Study the drawing (mm; zero at the part's minimum x, y, z) and answer. A direction names the side the tool comes from. Coordinates: 2 decimals unless noted, no trailing zeros. Order: outer loops, then holes, each group sorted by start corner. A loop starts at its lowest first (then second) coordinate and runs counter-clockwise, first axis right, second up.
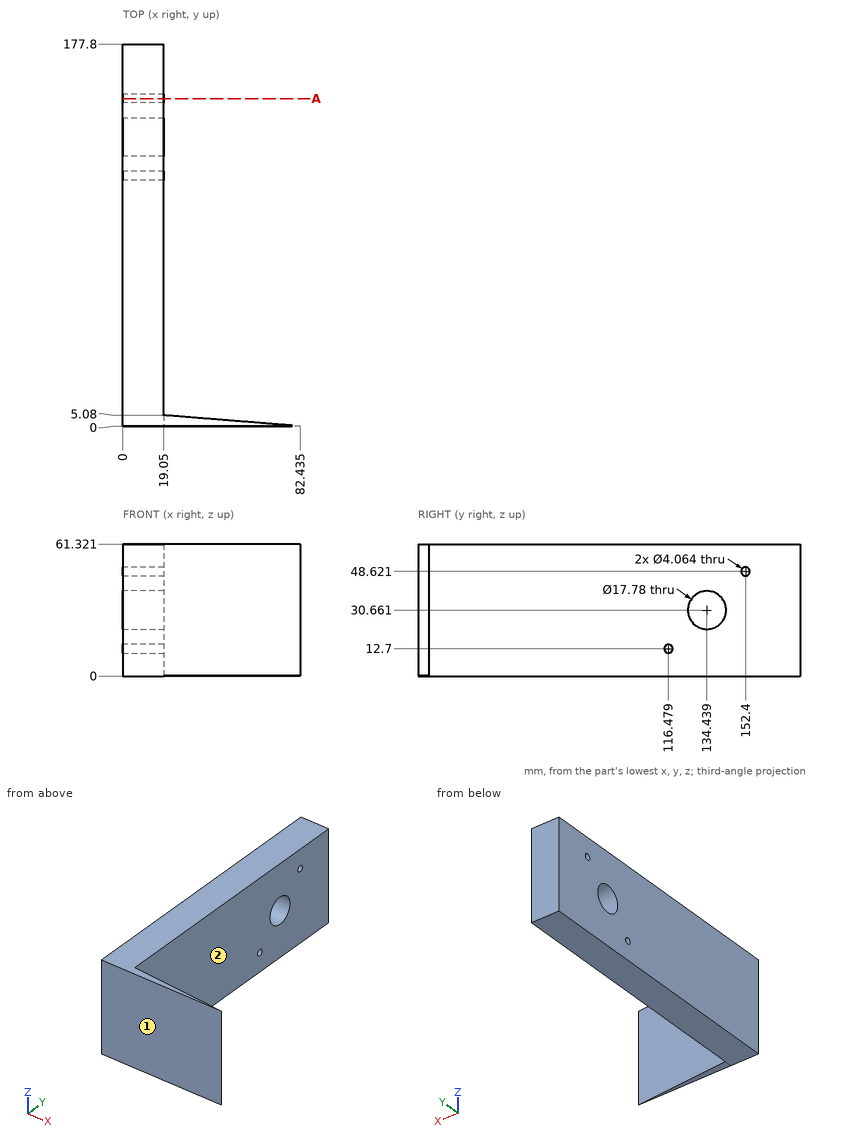
(1) Find section A-A (y = 152.4). Write down the section's boundary in (x, z).
(2) For the marked faces 1 and 2, determine the directions among +Z, -Z, +X, -X, +Y, -Y from which every point of the face is accessible in a straight line to the end or side of a thin tool.
(3) Each of these flat-tipped pins is pushed along its axis until it touches: pin 1 Ø4 at (x, z) = (67.5, 51) entering from -Y; pin 2 Ø3 at (x, z) = (43, 11.5) entering from +Y; pin 3 Ø4.5 at (y, z) = (152.4, 48.62) entering from +X. Where does it stop, or does it pass through?
(4) Consider line 1 (X direction, y = 91, z = 24); line 2 (Z direction, x = 11, y = 152); line 3 (Y direction, x = 4, z = 12) (1 decimal). Determine where each line is inside the solid, lowest interval first.
Findings below:
1. outline: (0, 0) - (19.05, 0) - (19.05, 46.59) - (0, 46.59) - close; (0, 50.65) - (19.05, 50.65) - (19.05, 61.32) - (0, 61.32) - close
2. face 1: +Z, -Z, +X, -X, -Y
2. face 2: +Z, -Z, +X, +Y
3. pin 1: stops at y = 0
3. pin 2: stops at y = 3.28
3. pin 3: stops at x = 19.05
4. line 1: x = 0 to 19.05
4. line 2: z = 0 to 46.63, 50.61 to 61.32
4. line 3: y = 0 to 114.6, 118.4 to 177.8
